Part model, mm, in its own coordinate system. Face numbers are marked on the shaded views. A direction names the side the tool comes from. Give positions to 0.01 mm unless a question says otherwise; leave off trailing zeros. Order: outer loops, then holes, each group sorted by start corner. A loop starts at its lowest first (then second) coordinate and runs counter-clockwise, first axis right, second up. Notation, with made-up numbers: (-32.75, -8.5) - (-28.75, -8.5) arc R26 ccw to (-28.75, 12.5) - close; hole circle Ø11 at (74.5, 71.25). An arc over 180 degrees is marked (long way). One line per item, written item: value.
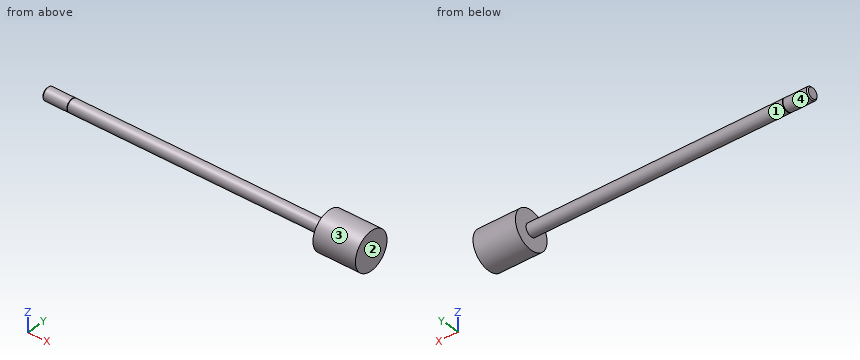
Autodesk Inventor part; units mm, degrees
ref_plane "dia1_XY" through (0, 3.175, 0) normal (1, 0, 0) x (0, 0, -1)
ref_plane "dia1_YZ" through (0, 3.175, 0) normal (0, 0, -1) x (0, 1, 0)
ref_plane "dia1_ZX" through (0, 3.175, 0) normal (0, 1, 0) x (1, 0, 0)
sketch "Sketch_1" plane through (0, 0, 0) normal (0, 0, 1) x (1, 0, 0)
  line L0 (150.8252, 0) -> (0, 0)
  line L1 (0, 0) -> (0, 3.175)
  line L2 (0, 3.175) -> (129.3876, 3.175)
  line L3 (129.3876, 3.175) -> (129.3876, 9.6203)
  line L4 (129.3876, 9.6203) -> (150.8252, 9.6203)
  line L5 (150.8252, 9.6203) -> (150.8252, 0)
  line L6 (150.8252, 0) -> (0, 0)
revolve "Revolution1" add sketch "Sketch_1" angle 360 about axis through (150.8252, 0, 0) along (1, 0, 0)
sketch "Sketch_3" plane through (0, 0, 0) normal (0, 0, 1) x (1, 0, 0)
  line L0 (0, 0) -> (-12.7, 0)
  line L1 (-12.7, 0) -> (-12.7, 2.634)
  line L2 (-12.7, 2.634) -> (-12.159, 3.175)
  line L3 (-12.159, 3.175) -> (0, 3.175)
  line L4 (0, 3.175) -> (0, 0)
  line L5 (0, 0) -> (-12.7, 0)
revolve "Revolution2" add sketch "Sketch_3" angle 360 about axis through (0, 0, 0) along (1, 0, 0)
thread "Thread1"
sketch "Sketch_30" plane through (0, 0, 0) normal (0, 0, 1) x (1, 0, 0)
  line L0 (0, 0) -> (-0.254, 0)
  line L1 (-0.254, 2.921) -> (0, 2.921)
  line L2 (0, 2.921) -> (0, 3.429)
  line L3 (0, 3.429) -> (-0.254, 3.429)
  line L4 (-0.254, 3.429) -> (-0.254, 2.921)
revolve "Revolution3" cut sketch "Sketch_30" angle 360 about axis through (0, 0, 0) along (1, 0, 0)
ref_plane "dia1_XY" through (0, 3.175, 0) normal (1, 0, 0) x (0, 0, -1)
ref_plane "dia1_YZ" through (0, 3.175, 0) normal (0, 0, -1) x (0, 1, 0)
ref_plane "dia1_ZX" through (0, 3.175, 0) normal (0, 1, 0) x (1, 0, 0)
ref_plane "dia12_XY" through (0, 0, 10.9537) normal (1, 0, 0) x (0, 0, -1)
ref_plane "dia12_YZ" through (0, 0, 10.9537) normal (0, 0, -1) x (0, 1, 0)
ref_plane "dia12_ZX" through (0, 0, 10.9537) normal (0, 1, 0) x (1, 0, 0)
ref_plane "dia2_XY" through (0, -3.175, 0) normal (1, 0, 0) x (0, 0, -1)
ref_plane "dia2_YZ" through (0, -3.175, 0) normal (0, 0, -1) x (0, 1, 0)
ref_plane "dia2_ZX" through (0, -3.175, 0) normal (0, 1, 0) x (1, 0, 0)
ref_plane "dia22_XY" through (0, 0, -10.9537) normal (1, 0, 0) x (0, 0, -1)
ref_plane "dia22_YZ" through (0, 0, -10.9537) normal (0, 0, -1) x (0, 1, 0)
ref_plane "dia22_ZX" through (0, 0, -10.9537) normal (0, 1, 0) x (1, 0, 0)
ref_plane "hh1_XY" through (180.9496, 0, 0) normal (0, 0, 1) x (1, 0, 0)
ref_plane "hh1_YZ" through (180.9496, 0, 0) normal (1, 0, 0) x (0, 1, 0)
ref_plane "hh1_ZX" through (180.9496, 0, 0) normal (0, 1, 0) x (0, 0, 1)
ref_plane "hh2_XY" through (187.3504, 0, 0) normal (0, 0, 1) x (1, 0, 0)
ref_plane "hh2_YZ" through (187.3504, 0, 0) normal (1, 0, 0) x (0, 1, 0)
ref_plane "hh2_ZX" through (187.3504, 0, 0) normal (0, 1, 0) x (0, 0, 1)
ref_plane "rl1_XY" through (-12.7, 0, 0) normal (1, 0, 0) x (0, 0, -1)
ref_plane "rl1_YZ" through (-12.7, 0, 0) normal (0, 0, -1) x (0, 1, 0)
ref_plane "rl1_ZX" through (-12.7, 0, 0) normal (0, 1, 0) x (1, 0, 0)
ref_plane "rl2_XY" through (0, 0, 0) normal (1, 0, 0) x (0, 0, -1)
ref_plane "rl2_YZ" through (0, 0, 0) normal (0, 0, -1) x (0, 1, 0)
ref_plane "rl2_ZX" through (0, 0, 0) normal (0, 1, 0) x (1, 0, 0)
ref_plane "rod_cp_XY" through (0, 0, 0) normal (1, 0, 0) x (0, 0, -1)
ref_plane "rod_cp_YZ" through (0, 0, 0) normal (0, 0, -1) x (0, 1, 0)
ref_plane "rod_cp_ZX" through (0, 0, 0) normal (0, 1, 0) x (1, 0, 0)
ref_plane "thd1_XY" through (-12.7, 3.175, 0) normal (1, 0, 0) x (0, 0, -1)
ref_plane "thd1_YZ" through (-12.7, 3.175, 0) normal (0, 0, -1) x (0, 1, 0)
ref_plane "thd1_ZX" through (-12.7, 3.175, 0) normal (0, 1, 0) x (1, 0, 0)
ref_plane "thd2_XY" through (-12.7, -3.175, 0) normal (1, 0, 0) x (0, 0, -1)
ref_plane "thd2_YZ" through (-12.7, -3.175, 0) normal (0, 0, -1) x (0, 1, 0)
ref_plane "thd2_ZX" through (-12.7, -3.175, 0) normal (0, 1, 0) x (1, 0, 0)
ref_plane "to_rod_clevis_XY" through (-16.764, 0, 0) normal (1, 0, 0) x (0, 0, -1)
ref_plane "to_rod_clevis_YZ" through (-16.764, 0, 0) normal (0, 0, -1) x (0, 1, 0)
ref_plane "to_rod_clevis_ZX" through (-16.764, 0, 0) normal (0, 1, 0) x (1, 0, 0)
properties part number "043.5-DXP0000_rod"
1) Cut at C-C, the plane x = 13. Give the cut face in (y, z) (3 decimals).
Outcome:
outline: circle Ø6.35 at (0, 0)
2) Pin check, flat tips, straight feed: pin 1 (4 mm diameter, centred on x = 28.5, y = -3.5, fed in from +Z); pin 2 (6 mm diameter, centred on y = -4.5, z = -3.5, fed in from -X); pin 3 (6 mm diameter, centred on x = 80.5, y = 1.5, fed in from +Z) (3 decimals); pin 4 (5 mm diameter, centred on x = 28, y = -6.5, fed in from +Z). Stop position of each tip, or through.
Outcome:
pin 1: stops at z = 2.8
pin 2: stops at x = -12.63
pin 3: stops at z = 3.175
pin 4: passes through
3) Drill centre lines: line 1 along X through (y, z) = (4.25, -2); line 2 along Y through (x, z) = (82, -2.5); line 3 along Z through (x, y) = (128, 1). Where is each one in solid material? Low to high. Write a range as from..to.
Outcome:
line 1: x = 129.39..150.83
line 2: y = -1.96..1.96
line 3: z = -3.01..3.01
4) Cut at A-A, the plane z = 0. Give the cut face in (x, y) (3 decimals).
Outcome:
outline: (-12.7, -2.634) - (-12.159, -3.175) - (-0.254, -3.175) - (-0.254, -2.921) - (0, -2.921) - (0, -3.175) - (129.388, -3.175) - (129.388, -9.62) - (150.825, -9.62) - (150.825, 9.62) - (129.388, 9.62) - (129.388, 3.175) - (0, 3.175) - (0, 2.921) - (-0.254, 2.921) - (-0.254, 3.175) - (-12.159, 3.175) - (-12.7, 2.634) - close
5) Mould opens along Z. For the marked faces 1 and 2 say: released by +Z, released by -Z, zero draft, split by the parting line, or undercut.
Outcome:
face 1: split by the parting line
face 2: zero draft
6) Which spindle directions (+Z, -Z, +X, -X, +Y, -Y) get a long thin tool onto all of the face, cutting with end or side? Do the marked faces 3 and 4. Say none if no direction does.
Outcome:
face 3: +X, -X
face 4: -X
7) Cut at D-D, the plane z = 6.5. Give the cut face in (x, y), then the cut area to 3 significant figures.
Outcome:
outline: (129.39, -7.09) - (150.83, -7.09) - (150.83, 7.09) - (129.39, 7.09) - close
area: 304 mm^2
